```python
from build123d import *

# Parameters (mm, degrees)
F0_R     = 14.224
F1_DEPTH = 50.8
F3_DEPTH = 177.8
F4_R     = 7.874
F5_DEPTH = 25.4


with BuildPart() as f1:
    # F0 (on Front) → F1 (new body)
    with BuildSketch(Plane.XZ):
        Polygon((-32.6052582374, 11.9092461534), (-70.7052582374, 11.9092461534), (-70.7052582374, -0.7907538466), (62.3907417626, -0.7907538466), (62.3907417626, 11.9092461534), (24.2907417626, 11.9092461534), align=None)
        with BuildLine():
            Line((-32.6052582374, 14.9572461534), (-32.6052582374, 11.9092461534))
            Line((-32.6052582374, 11.9092461534), (24.2907417626, 11.9092461534))
            Line((24.2907417626, 11.9092461534), (24.2907417626, 14.9572461534))
            Line((24.2907417626, 14.9572461534), (24.2907417626, 40.3572461534))
            ThreePointArc((24.2907417626, 40.3572461534), (-4.1572582374, 68.8052461534), (-32.6052582374, 40.3572461534))
            Line((-32.6052582374, 40.3572461534), (-32.6052582374, 14.9572461534))
        make_face()
        with Locations((-4.1572582374, 40.3572461534)):
            Circle(F0_R, mode=Mode.SUBTRACT)
    extrude(amount=F1_DEPTH)

    # F2 (on face) → F3 (cut)
    with BuildSketch(Plane.YZ.offset(24.2907417626)):
        Polygon((-50.8, 68.8053369522), (-30.0915165031, 68.8053369522), (-28.7422632826, 72.5123797086), (-50.8, 72.5123797086), align=None)
        Polygon((-50.8, 40.3572461534), (-50.8, 11.9092461534), (-40.4457747756, 40.3572461534), align=None)
        Polygon((-50.8, 40.3572461534), (-40.4457747756, 40.3572461534), (-30.0915165031, 68.8053369522), (-50.8, 68.8053369522), align=None)
    extrude(amount=-F3_DEPTH, mode=Mode.SUBTRACT)

    # F4 (on face) → F5 (cut)
    with BuildSketch(Plane.XY.offset(11.9092461534)):
        with Locations((-49.8867883899, -25.4)):
            Circle(F4_R)
        with Locations((45.6172116101, -25.4)):
            Circle(F4_R)
    extrude(amount=-F5_DEPTH, mode=Mode.SUBTRACT)


solid = f1.part
```
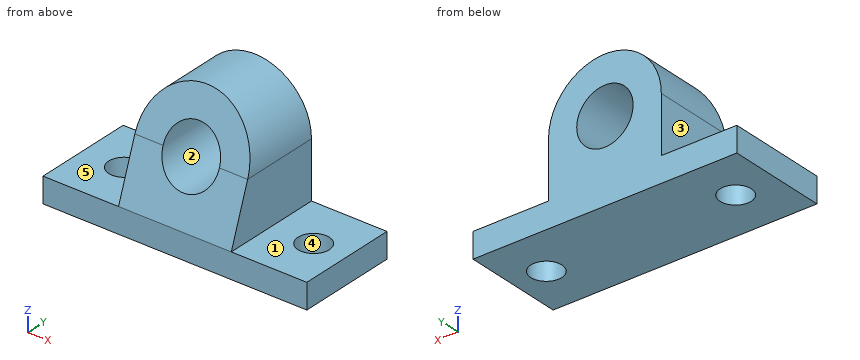
Can you work these out from the model? Positions are in its coordinate system, mm. Face numbers are marked on the shaded views. A direction names the side the tool comes from. Coordinates: 2 decimals unless noted, no trailing zeros. Write each loop counter-clockwise with the first axis right and the second up, starting at its lowest first coordinate (ties: lowest second). Pieces come first, ordered by that corner, then holes. Notation, with made-up numbers: M 68,13 L 91,13 A19 ccw 91,23 Z; hole C -10.75,14 d6. An arc over 180 degrees is marked long. Write item = value, one per line. Start each with the question number.
Q1. On a 3-axis mill with a long thin cutter (end or side, diameter ignored), from which of +Z, -Z, +X, -X, +Y, -Y can I reach the whole of each face in a straight line? I mean the marked faces 1 and 2. Say none if no direction works.
Q2. If I drill on L1, parallel to X at y = -25, z = 5; L2, parallel to Z at x = -48, y = -47.5; L3, parallel to X at y = -35, z = 24.5, over which ranges is the centre line in solid material (lowest first)? Write a range as [from, to].
Q3. If we section it at D-D, the plane z = 51.5: Write out the boundary of the cut face in (x, y).
Q4. Thinking about a two-plate mould opening in X: for the marked faces 3, 4 and 5, which applies, released by +X, released by -X, zero draft, split by the parting line, or undercut?
Q5. I'm going to push flat-ended pins straight in: pin 1 (4 mm diameter, centred on x = 37.5, y = -5.5, fed in from +Z); pin 2 (20.5 mm diameter, centred on x = 45.62, y = -25.4, fed in from -Z); pin 3 (8 mm diameter, centred on y = -20, z = 20.5, fed in from +X); pin 4 (10 mm diameter, centred on x = 22, y = -30, fed in from +Z). Where does each tip first touch, or does it pass through?
Q6. If we section it at A-A, the plane y = -25.4: Write out the boundary of the cut face in (x, z).
Q7. If we section it at C-C, the plane x = 0: Write out the boundary of the cut face in (y, z).
Q8. If we section it at B-B, the plane z = 33: Write out the boundary of the cut face in (x, y), then the cut area to 3 significant figures.
Check sheet entries:
q1.face_1 = +Z, +X, +Y, -Y
q1.face_2 = +Y, -Y
q2.L1 = [-70.71, -57.75], [-42.02, 37.75], [53.48, 62.39]
q2.L2 = [-0.79, 11.91]
q2.L3 = [-32.61, 24.29]
q3.outline = M -30.33,-36.39 L -13,-36.39 L -13,0 L -30.33,0 Z; M 4.68,-36.39 L 22.02,-36.39 L 22.02,0 L 4.68,0 Z
q4.face_3 = released by -X
q4.face_4 = undercut
q4.face_5 = zero draft
q5.pin_1 = 11.91
q5.pin_2 = -0.79
q5.pin_3 = 24.29
q5.pin_4 = 59.37
q6.outline = M -70.71,-0.79 L -57.76,-0.79 L -57.76,11.91 L -70.71,11.91 Z; M -42.01,-0.79 L 37.74,-0.79 L 37.74,11.91 L 24.29,11.91 L 24.29,40.36 A28.45 ccw -32.61,40.36 L -32.61,11.91 L -42.01,11.91 Z; M 53.49,-0.79 L 62.39,-0.79 L 62.39,11.91 L 53.49,11.91 Z; hole C -4.16,40.36 d28.45
q7.outline = M -50.8,-0.79 L 0,-0.79 L 0,26.75 L -45.4,26.75 L -50.8,11.91 Z; M -35.49,53.96 L 0,53.96 L 0,68.5 L -30.2,68.5 Z
q8.outline = M -32.61,-43.12 L -16.33,-43.12 L -16.33,0 L -32.61,0 Z; M 8.02,-43.12 L 24.29,-43.12 L 24.29,0 L 8.02,0 Z
q8.area = 1,400 mm²
